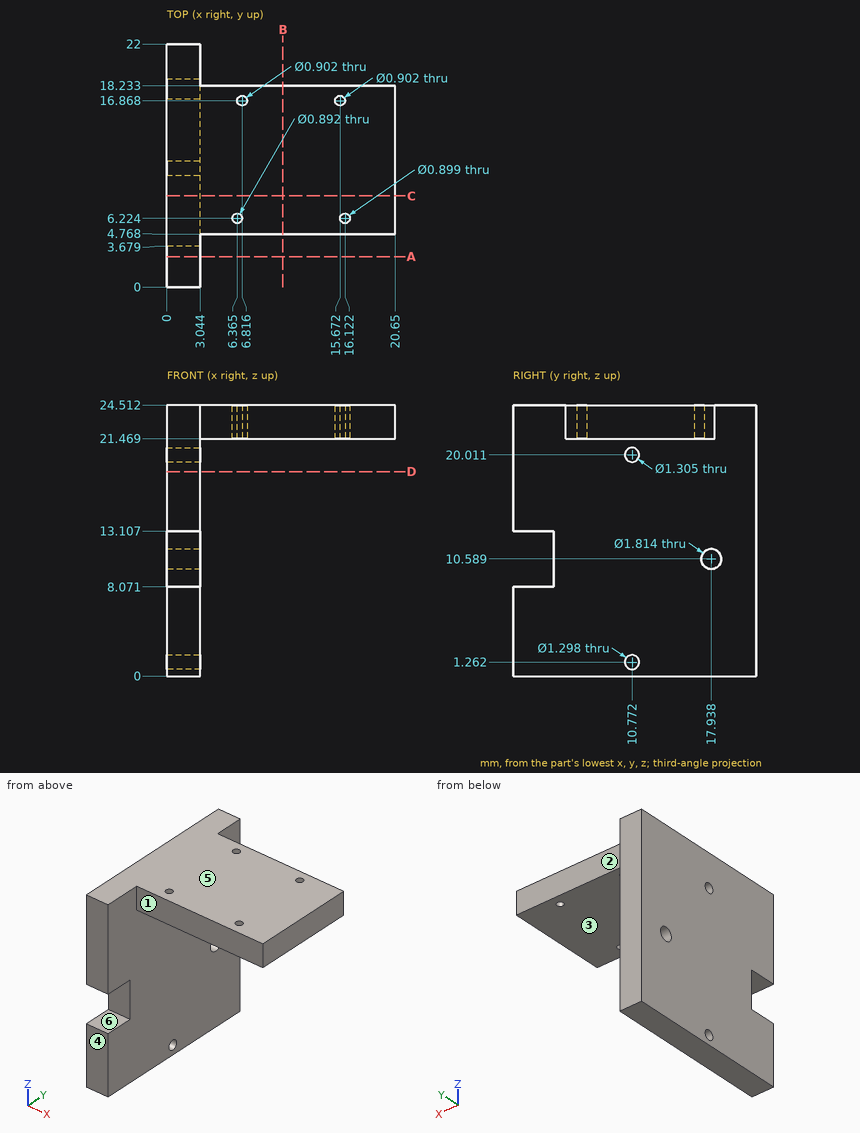
Part print with two shaded views. Sizes in mm from the minimum x, y, z corner. A direction names the side the tool comes from. Coordinates: 2 decimals unless noted, no trailing zeros. Order: outer loops, then holes, each group sorted by start corner. A loop starts at its lowest first (then second) coordinate and runs counter-clockwise, first axis right, second up. Notation, with made-up numbers: M 31.5,-28.5 L 36.5,-28.5 A16 cw 36.5,-12.5 Z; hole C 14.5,-20.5 d7. An arc over 180 degrees is marked long. One line per question, with ' | ' between items. Start each with the question number.
1. Flat gauge pins, fed straight in: P1, Ø1.5, axis at x = 10, z = 23.5, coming from the +Y side; P2, Ø1.5, axis at x = 1.5, z = 10, coming from the -Y side; P3, Ø6.5, axis at y = 7.5, z = 6.5, coming from the +X side; P4, Ø0.8, axis at y = 10.77, z = 1.26, coming from the -X side. Where does each tip first touch, or does it go through?
2. Tool access for the marked faces 1, 2 and 3: list every direction of +Z, -Z, +X, -X, +Y, -Y with a clear straight run to the whole face (end or side of a thin tool).
3. Mould opens along Z. For the marked faces 4, 5 and 6 say: +Z half, -Z half, draft (parallel to the pull), parting line (faces both ways), or undercut.
4. Cut at C-C (y = 8.25). Write the cut outline in (x, z).
5. Cut at A-A (y = 2.75). Write the cut outline in (x, z).
6. Cut at D-D (z = 18.5). Write the cut outline in (x, y).
7. Cut at B-B (x = 10.5). Write the cut outline in (y, z).
8. Wall check: line 1 along X through (y, z) = (12.5, 17.25); line 2 along Z through (x, y) = (19, 17.5); line 3 along Y through (x, z) = (16.25, 23) (1 decimal). Give the ranges that are in metal, low to high. Write a range as [from, to].
The answers:
1) P1: stops at y = 18.23 | P2: stops at y = 3.68 | P3: stops at x = 3.04 | P4: passes through
2) face 1: +Z, -Z, +X, -Y | face 2: +Z, -Z, +X, +Y | face 3: -Z, +X, +Y, -Y
3) face 4: draft | face 5: +Z half | face 6: undercut
4) outline: M 0,0 L 3.04,0 L 3.04,21.47 L 20.65,21.47 L 20.65,24.51 L 0,24.51 Z
5) outline: M 0,0 L 3.04,0 L 3.04,8.07 L 0,8.07 Z; M 0,13.11 L 3.04,13.11 L 3.04,24.51 L 0,24.51 Z
6) outline: M 0,0 L 3.04,0 L 3.04,22 L 0,22 Z
7) outline: M 4.77,21.47 L 18.23,21.47 L 18.23,24.51 L 4.77,24.51 Z
8) line 1: x = [0, 3.04] | line 2: z = [21.47, 24.51] | line 3: y = [4.8, 5.8], [6.7, 18.2]
